```python
from build123d import *

# Parameters (mm, degrees)
SKETCH_1_W      = 64
SKETCH_1_H      = 42
SKETCH_1_R      = 1.5
EXTRUDE_1_DEPTH = 3
FILLET_2_R      = 5


with BuildPart() as part:
    # 草图1 → 凸台-拉伸1 (new body)
    with BuildSketch(Plane(origin=(0, 0, 0), x_dir=(1, 0, 0), z_dir=(0, 1, 0))):
        with Locations((0, -5)):
            Rectangle(SKETCH_1_W, SKETCH_1_H)
        with Locations(Location((-27.5, -10, 0), (0, 0, 270))):
            Circle(SKETCH_1_R, mode=Mode.SUBTRACT)
        with Locations(Location((-12, -13, 0), (0, 0, 270))):
            Circle(SKETCH_1_R, mode=Mode.SUBTRACT)
        with Locations(Location((12, -13, 0), (0, 0, 270))):
            Circle(SKETCH_1_R, mode=Mode.SUBTRACT)
        with Locations(Location((27.5, -10, 0), (0, 0, 270))):
            Circle(SKETCH_1_R, mode=Mode.SUBTRACT)
        with Locations(Location((-24.75, 3, 0), (0, 0, 270))):
            Circle(SKETCH_1_R, mode=Mode.SUBTRACT)
        with Locations(Location((-27.5, 12, 0), (0, 0, 270))):
            Circle(SKETCH_1_R, mode=Mode.SUBTRACT)
        with Locations(Location((-12, 13, 0), (0, 0, 270))):
            Circle(SKETCH_1_R, mode=Mode.SUBTRACT)
        with Locations(Location((24.75, 3, 0), (0, 0, 270))):
            Circle(SKETCH_1_R, mode=Mode.SUBTRACT)
        with Locations(Location((12, 13, 0), (0, 0, 270))):
            Circle(SKETCH_1_R, mode=Mode.SUBTRACT)
        with Locations(Location((27.5, 12, 0), (0, 0, 270))):
            Circle(SKETCH_1_R, mode=Mode.SUBTRACT)
        with Locations(Location((24.75, -23, 0), (0, 0, 270))):
            Circle(SKETCH_1_R, mode=Mode.SUBTRACT)
        with Locations(Location((-24.75, -23, 0), (0, 0, 270))):
            Circle(SKETCH_1_R, mode=Mode.SUBTRACT)
    extrude(amount=EXTRUDE_1_DEPTH)

    # 圆角2
    fillet_2_edges = [part.edges().sort_by_distance(p)[0] for p in [
        (-32, 1.5, -16),
        (32, 1.5, -16),
        (32, 1.5, 26),
        (-32, 1.5, 26),
    ]]
    fillet(fillet_2_edges, radius=FILLET_2_R)


solid = part.part
```
Read the model definition and answer for the solid it produces. Units are mm, in the model's axes. Coordinates: 2 decimals unless noted, no trailing zeros. Loops run counter-clockwise (first coordinate to the right, second up) from the corner with the lowest first, then second, coordinate; pieces in that order, holes last. Notation, with made-up numbers: (68, 24.25) -> (94, 24.25) arc R17 ccw to (94, 34.25) -> close; hole circle Ø8 at (63, 37). An arc over 180 degrees is marked (long way). Return JSON: item names as keys, results as strings.
Item 1: Flat-ended cylindrical pins translate along their axes: P1, Ø3.5, axis at x = -27.5, z = 10, coming from the -Y side; P2, Ø2.5, axis at x = 24.75, z = 23, coming from the +Y side. Find the tip coordinate at first contact, or state that the pin passes through.
Answers:
{"P1": "stops at y = 0", "P2": "passes through"}
Item 2: Find the intervals of material crossed by probe 1 along X at (y, z) = (0.8, 10); probe 2 along X at (y, z) = (0.9, 13); probe 3 along X at (y, z) = (1.45, -12), in increasing order.
Answers:
{"probe 1": "x = -32 to -29, -26 to 26, 29 to 32", "probe 2": "x = -32 to -13.5, -10.5 to 10.5, 13.5 to 32", "probe 3": "x = -31.9 to -29, -26 to -13.12, -10.88 to 10.88, 13.12 to 26, 29 to 31.9"}
Item 3: Find section B-B (y = 0.5). Count the separate pieces of the cut face and the enclosed holes in it, plus the area to 3 significant figures.
Answers:
{"separate pieces": "1", "enclosed holes": "12", "area": "2,580 mm2"}
Item 4: For a pull along X with two mould halves and no side action, classify faces 1 (the cylindrical face through (-31, 2, 24)), 2 (the cylindrical face through (30, 2, 25)), 3 (the cylindrical face through (-23.263, 1.479, 22.805)), 4 (the cylindrical face through (12.07, 1.48, 11.5)) as +X half, -X half, draft (parallel to the pull), parting line (faces both ways), or undercut.
Answers:
{"face 1": "-X half", "face 2": "+X half", "face 3": "undercut", "face 4": "undercut"}
Item 5: Find section C-C (x = 24.75). Determine the outline of the cut face in (y, z).
Answers:
{"outline": "(0, -16) -> (3, -16) -> (3, -4.5) -> (0, -4.5) -> close; (0, -1.5) -> (3, -1.5) -> (3, 21.5) -> (0, 21.5) -> close; (0, 24.5) -> (3, 24.5) -> (3, 26) -> (0, 26) -> close"}
Item 6: Find section A-A (z = -3). Determine the outline of the cut face in (x, y), plus the area to 3 significant figures.
Answers:
{"outline": "(-32, 0) -> (-26.25, 0) -> (-26.25, 3) -> (-32, 3) -> close; (-23.25, 0) -> (23.25, 0) -> (23.25, 3) -> (-23.25, 3) -> close; (26.25, 0) -> (32, 0) -> (32, 3) -> (26.25, 3) -> close", "area": "174 mm2"}
